Geometry: final body of the model. Coordinates: model frame, mm. A direction names the side the tool comes from. Give positions to 0.01 mm unless a question says otherwise; leave off trailing zeros. Order: outer loops, then holes, each group sorted by start corner. A loop starts at its lowest first (then second) coordinate and runs counter-clockwise, first axis right, second up. Notation, with made-up numbers: (-37, 14) -> (-25, 14) arc R12 cw to (-25, 29) -> close; hole circle Ø4 at (-23, 38.5). An arc over 180 degrees is marked (long way). One line per question, with ' | ' between items.
from build123d import *

# Parameters (mm, degrees)
BOSS_EXTRUDE1_DEPTH       = 15
M4X0_7_TAPPED_HOLE1_D     = 3.3
M4X0_7_TAPPED_HOLE1_DEPTH = 8
M4X0_7_TAPPED_HOLE1_TIP   = 0.991420021
F_3_0MM_DOWEL_HOLE1_D     = 3
F_3_0MM_DOWEL_HOLE1_DEPTH = 4.85
F_3_0MM_DOWEL_HOLE1_TIP   = 0.901290929
SKETCH6_R                 = 14
CUT_EXTRUDE1_DEPTH        = 30


with BuildPart() as part:
    # Sketch1 → Boss-Extrude1 (new, symmetric)
    with BuildSketch(Plane(origin=(0, 0, 0), x_dir=(1, 0, 0), z_dir=(0, 1, 0))):
        with BuildLine():
            Line((13.266499161, 20), (-13.266499161, 20))
            ThreePointArc((-13.266499161, 20), (-21.147056295, 11.349097324), (-24, 0))
            Line((-24, 0), (-24, -24))
            Line((-24, -24), (24, -24))
            Line((24, -24), (24, 0))
            ThreePointArc((24, 0), (21.147056295, 11.349097324), (13.266499161, 20))
        make_face()
    extrude(amount=BOSS_EXTRUDE1_DEPTH, both=True)

    # M4x0.7 Tapped Hole1
    with Locations(Plane.XY.offset(24)):
        with Locations((-19.86, 9.95), (0, 9.95), (19.86, 9.95), (19.86, -9.95), (0, -9.95), (-19.86, -9.95)):
            Hole(M4X0_7_TAPPED_HOLE1_D / 2, depth=M4X0_7_TAPPED_HOLE1_DEPTH)
            with Locations((0, 0, -(M4X0_7_TAPPED_HOLE1_DEPTH + M4X0_7_TAPPED_HOLE1_TIP / 2))):  # 118° drill point
                Cone(0, M4X0_7_TAPPED_HOLE1_D / 2, M4X0_7_TAPPED_HOLE1_TIP, mode=Mode.SUBTRACT)

    # 3.0mm Dowel Hole1
    with Locations(Plane.XY.offset(24)):
        with Locations((-17.5, 0), (17.5, 0)):
            Hole(F_3_0MM_DOWEL_HOLE1_D / 2, depth=F_3_0MM_DOWEL_HOLE1_DEPTH)
            with Locations((0, 0, -(F_3_0MM_DOWEL_HOLE1_DEPTH + F_3_0MM_DOWEL_HOLE1_TIP / 2))):  # 118° drill point
                Cone(0, F_3_0MM_DOWEL_HOLE1_D / 2, F_3_0MM_DOWEL_HOLE1_TIP, mode=Mode.SUBTRACT)

    # Sketch6 → Cut-Extrude1 (cut)
    with BuildSketch(Plane.XZ.offset(15)):
        with Locations(Location((0, 0, 0), (0, 0, 270))):
            Circle(SKETCH6_R)
    extrude(amount=-CUT_EXTRUDE1_DEPTH, mode=Mode.SUBTRACT)


solid = part.part
1) Set-up query: faces 1 (the flat face through (0, 0, -20)), 2 (the cylindrical face through (18.286, 10.446, 19.944)). Return all of +Z, -Z, +X, -X, +Y, -Y with unobstructed straight access to the full face (end or side cutting, diameter ignored); none if empty.
Check result:
face 1: -Z, +X, -X, +Y, -Y | face 2: +Z
2) Contact query for flat-ended pins moving along their axis: pin 1 Ø2 at (y, z) = (1.5, -15) entering from -X; pin 2 Ø12 at (x, z) = (1.5, 12) entering from -Y; pin 3 Ø5.5 at (x, y) = (19.86, 9.95) entering from -Z; pin 4 Ø6 at (y, z) = (3.5, -13) entering from +X. Output: stop coordinate, or through.
Check result:
pin 1: stops at x = -19.49 | pin 2: stops at y = -15 | pin 3: stops at z = -16.83 | pin 4: stops at x = 21.82
3) Pull-direction query (X, two-part tool) for faces 3 (the flat face through (0, 15, 16)), 4 (the cylindrical face through (-21.07, 0.21, -11.49)), 5 (the cylindrical face through (0.215, -8.314, 19.944)); classes: +X half, -X half, draft (parallel to the pull), parting line (faces both ways), or undercut.
Check result:
face 3: draft | face 4: -X half | face 5: undercut
4) Section C-C on x = -9. Return loops of the section in (y, z), plus the area to 3 significant figures.
Check result:
outline: (-15, -20) -> (15, -20) -> (15, -10.72) -> (-15, -10.72) -> close; (-15, 10.72) -> (15, 10.72) -> (15, 24) -> (-15, 24) -> close | area: 677 mm^2
5) Section A-A on y = -5.5. Return loops of the section in (x, z).
Check result:
outline: (-24, 0) arc R24 ccw to (-13.27, -20) -> (13.27, -20) arc R24 ccw to (24, 0) -> (24, 24) -> (-24, 24) -> close; hole circle Ø28 at (0, 0)
6) Material intervals for probe 1 along Y at (x, z) = (19.86, 20); probe 2 along X at (y, z) = (0, 21.9); probe 3 along X at (y, z) = (9.95, 19.5), sorted ascending. Write a range as from..to.
Check result:
probe 1: y = -15..-11.6, -8.3..8.3, 11.6..15 | probe 2: x = -24..-19, -16..16, 19..24 | probe 3: x = -24..-21.51, -18.21..-1.65, 1.65..18.21, 21.51..24
7) Section B-B on z = -1.5. Return loops of the section in (x, y).
Check result:
outline: (-23.95, -15) -> (-13.92, -15) -> (-13.92, 15) -> (-23.95, 15) -> close; (13.92, -15) -> (23.95, -15) -> (23.95, 15) -> (13.92, 15) -> close
